The drawing under review shows one solid part. Ordinate dimensions are in mm from its lowest x, y, z. A direction names the side the tool comes from. Give positions to 0.01 mm unless a question says otherwise; leave off trailing zeros. Loops run counter-clockwise (first coordinate to the right, second up) from the corner with the lowest first, then second, coordinate; pieces in that order, holes last. Notation, with made-up numbers: (-12.5, 60) - (31.5, 60) arc R18 ccw to (31.5, 69) - close; hole circle Ø4 at (-20, 77). An arc over 180 degrees is marked (long way). Write each question's results on one line, items separated by ' | '.
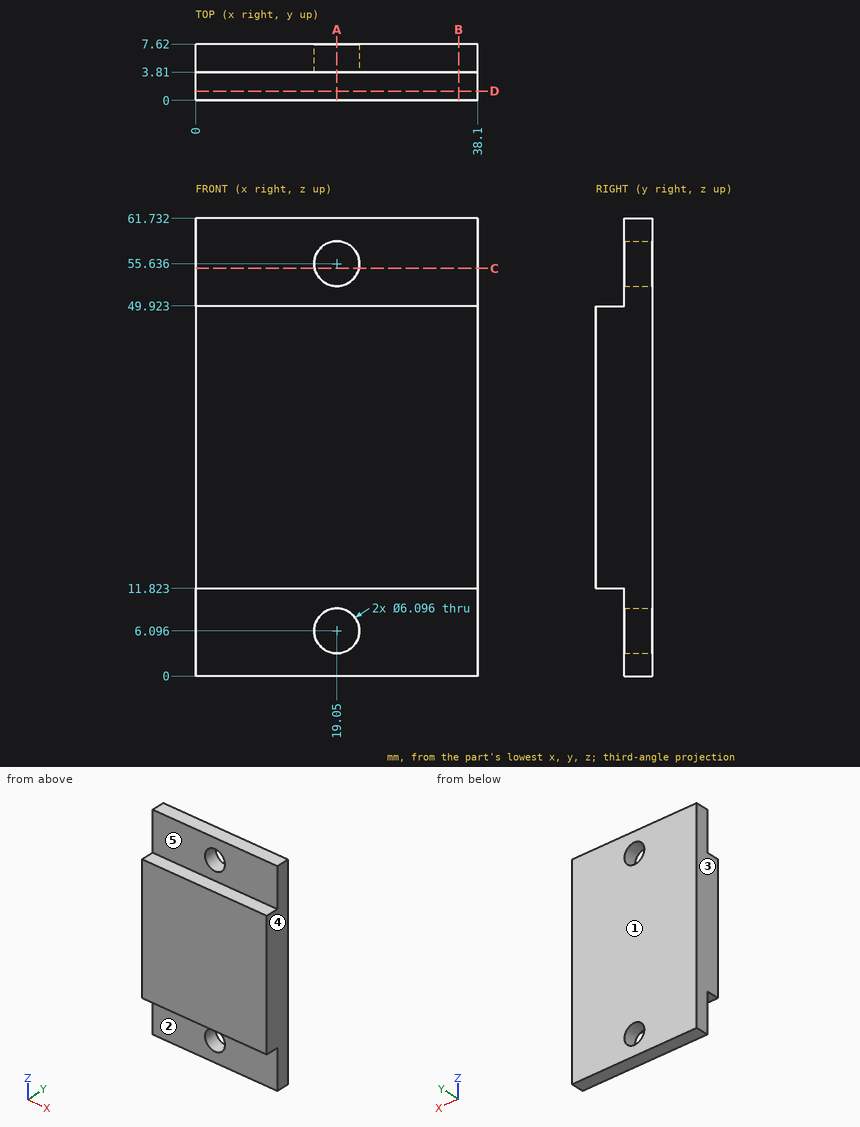
(1) Take a section at D-D on y = 1.25. Give the boundary of the cut face in (x, z), plus the area to 3 significant figures.
Answers below:
outline: (0, 11.82) - (38.1, 11.82) - (38.1, 49.92) - (0, 49.92) - close | area: 1,450 mm2
(2) Take a section at B-B on x = 35.5. Give the boundary of the cut face in (y, z), plus the area to 3 significant figures.
Answers below:
outline: (0, 11.82) - (3.81, 11.82) - (3.81, 0) - (7.62, 0) - (7.62, 61.73) - (3.81, 61.73) - (3.81, 49.92) - (0, 49.92) - close | area: 380 mm2
(3) Insertion check: P1, Ø1.5, axis at y = 2.5, z = 8.5, coming from the +X side; P2, Ø3.5, axis at x = 23.5, z = 7.5, coming from the -Y side. Each pin has a flat end and moves straight along its axis. Give the tip position at first contact, or say it passes through.
Answers below:
P1: through | P2: y = 3.81
(4) Wall thickness on line 1 along Z through (x, y) = (19.05, 6.2) (1 decimal); line 2 along Y through (x, z) = (15.5, 51); line 3 along Z through (x, y) = (14, 3.25): over which ranges is each line inside the solid? List them lowest first. Write a range as from..to.
Answers below:
line 1: 0..3, 9.1..52.6, 58.7..61.7 | line 2: 3.81..7.62 | line 3: 11.82..49.92
(5) Take a section at C-C on z = 55. Give the boundary of the cut face in (x, y).
Answers below:
outline: (0, 3.81) - (16.07, 3.81) - (16.07, 7.62) - (0, 7.62) - close; (22.03, 3.81) - (38.1, 3.81) - (38.1, 7.62) - (22.03, 7.62) - close
(6) Take a section at A-A on x = 19.05. Give the boundary of the cut face in (y, z) (1 decimal), plus the area to 3 significant figures.
Answers below:
outline: (0, 11.8) - (3.8, 11.8) - (3.8, 9.1) - (7.6, 9.1) - (7.6, 52.6) - (3.8, 52.6) - (3.8, 49.9) - (0, 49.9) - close; (3.8, 0) - (7.6, 0) - (7.6, 3) - (3.8, 3) - close; (3.8, 58.7) - (7.6, 58.7) - (7.6, 61.7) - (3.8, 61.7) - close | area: 334 mm2
(7) Draft analysis for pull direction Y (two halves, no side actions). For the marked faces 1, 2 and 3, state which applies: pulls with the +Y half, pulls with the -Y half, needs draft (parallel to the pull), parting line crosses it, or undercut.
Answers below:
face 1: pulls with the +Y half | face 2: pulls with the -Y half | face 3: needs draft
(8) Tool access review of the marked faces 4 and 5: name each direction out of +Z, -Z, +X, -X, +Y, -Y from which nothing blocks a thin tool from reaching the whole face with its end or side.
Answers below:
face 4: +Z, -Z, +X, +Y, -Y | face 5: +Z, +X, -X, -Y
